from build123d import *

# Parameters (mm, degrees)
BOSS_EXTRUDE1_DEPTH = 2.2
SKETCH3_R           = 7.5
BOSS_EXTRUDE2_DEPTH = 2
BOSS_EXTRUDE3_DEPTH = 2.5
SKETCH5_W           = 12
SKETCH5_H           = 11
CUT_EXTRUDE1_DEPTH  = 7.7
SKETCH6_W           = 40
SKETCH6_H           = 20
SKETCH6_W_2         = 12
SKETCH6_H_2         = 11
BOSS_EXTRUDE4_DEPTH = 3
SKETCH7_R           = 1.75
CUT_EXTRUDE2_DEPTH  = 10.7
SKETCH8_R           = 3
CUT_EXTRUDE3_DEPTH  = 1.5
SKETCH9_W           = 40
SKETCH9_H           = 2.5
CUT_EXTRUDE4_DEPTH  = 10.7


with BuildPart() as part:
    # Sketch2 → Boss-Extrude1 (new body)
    with BuildSketch(Plane.XY):
        with BuildLine():
            Line((-5.830951895, -7.5), (5.830951895, -7.5))
            ThreePointArc((5.830951895, -7.5), (0, 9.5), (-5.830951895, -7.5))
        make_face()
    extrude(amount=-BOSS_EXTRUDE1_DEPTH)

    # Sketch3 → Boss-Extrude2 (add)
    with BuildSketch(Plane(origin=(0, 0, -2.2), x_dir=(-1, 0, 0), z_dir=(0, 0, -1))):
        Circle(SKETCH3_R)
    extrude(amount=BOSS_EXTRUDE2_DEPTH)

    # Sketch4 → Boss-Extrude3 (add)
    with BuildSketch(Plane(origin=(0, 0, -4.2), x_dir=(-1, 0, 0), z_dir=(0, 0, -1))):
        with BuildLine():
            Line((-5.830951895, -7.5), (5.830951895, -7.5))
            ThreePointArc((5.830951895, -7.5), (0, 9.5), (-5.830951895, -7.5))
        make_face()
    extrude(amount=BOSS_EXTRUDE3_DEPTH)

    # Sketch5 → Cut-Extrude1 (cut, through all)
    with BuildSketch(Plane(origin=(0, 0, -6.7), x_dir=(-1, 0, 0), z_dir=(0, 0, -1))):
        Rectangle(SKETCH5_W, SKETCH5_H)
    extrude(amount=-CUT_EXTRUDE1_DEPTH, mode=Mode.SUBTRACT)

    # Sketch6 → Boss-Extrude4 (add)
    with BuildSketch(Plane.XY):
        Rectangle(SKETCH6_W, SKETCH6_H)
        Rectangle(SKETCH6_W_2, SKETCH6_H_2, mode=Mode.SUBTRACT)
    extrude(amount=BOSS_EXTRUDE4_DEPTH)

    # Sketch7 → Cut-Extrude2 (cut, through all)
    with BuildSketch(Plane.XY.offset(3)):
        with Locations((-15, 0)):
            Circle(SKETCH7_R)
        with Locations((15, 0)):
            Circle(SKETCH7_R)
    extrude(amount=-CUT_EXTRUDE2_DEPTH, mode=Mode.SUBTRACT)

    # Sketch8 → Cut-Extrude3 (cut)
    with BuildSketch(Plane(origin=(0, 0, 0), x_dir=(-1, 0, 0), z_dir=(0, 0, -1))):
        with Locations((15, 0)):
            Circle(SKETCH8_R)
        with Locations((-15, 0)):
            Circle(SKETCH8_R)
    extrude(amount=-CUT_EXTRUDE3_DEPTH, mode=Mode.SUBTRACT)

    # Sketch9 → Cut-Extrude4 (cut, through all)
    with BuildSketch(Plane(origin=(0, 0, -6.7), x_dir=(-1, 0, 0), z_dir=(0, 0, -1))):
        with Locations((0, -8.75)):
            Rectangle(SKETCH9_W, SKETCH9_H)
    extrude(amount=-CUT_EXTRUDE4_DEPTH, mode=Mode.SUBTRACT)


solid = part.part
Verification items for the finished model (mm, model axes). A direction names the side the tool comes from. Give positions to 0.01 mm unless a question says otherwise; leave off trailing zeros. Loops run counter-clockwise (first coordinate to the right, second up) from the corner with the lowest first, then second, coordinate; pieces in that order, holes last.
1. Cross-section at D-D on y = 0. Count the separate pieces of the cut face and the enclosed holes in it, and give its area (3 significant figures).
Derived:
separate pieces: 4
enclosed holes: 0
area: 94.4 mm2
2. Release check for a two-part mould opening along Y. For faces 1 (the cylindrical face through (-0.1, 7.5, -3.2)), 2 (the cylindrical face through (0.33, 9.494, -1.085)), 3 (the flat face through (6, 0, -2)) record: +Y half, -Y half, draft (parallel to the pull), parting line (faces both ways), or undercut.
Derived:
face 1: +Y half
face 2: parting line
face 3: undercut
3. Tool access check on faces 4 (the cylindrical face through (0.1, -7.5, -3.2)), 5 (the flat face through (0, 5.5, -2)), 6 (the cylindrical face through (7.5, 0.1, -3.2)), 7 (the flat face through (13, 0, 1.5)). Record the directions out of +Z, -Z, +X, -X, +Y, -Y that give a thin tool (end or side, any length) a straight path to the whole face; none if there is none.
Derived:
face 4: -Y
face 5: +Z, -Z
face 6: +X
face 7: -Z
4. Go/stop test with flat-tipped pins: P1, Ø4.5, axis at x = -15, y = 0, coming from the -Z side; P2, Ø7, axis at x = -15, y = 0, coming from the +Z side; P3, Ø1.5, axis at y = -1.5, z = -3.5, coming from the -X side; P4, Ø6.5, axis at x = 15, y = -0.5, coming from the -Z side. Record where each tip stops, or that it passes through.
Derived:
P1: stops at z = 1.5
P2: stops at z = 3
P3: stops at x = -9.42
P4: stops at z = 0
5. Cross-section at C-C on z = 2.5. Record the cut outline in (x, y).
Derived:
outline: (-20, -7.5) - (20, -7.5) - (20, 10) - (-20, 10) - close; hole circle Ø3.5 at (-15, 0); hole (-6, -5.5) - (6, -5.5) - (6, 5.5) - (-6, 5.5) - close; hole circle Ø3.5 at (15, 0)
6. Cross-section at B-B on y = 8. Record the cut outline in (x, z), and give its area (3 significant figures).
Derived:
outline: (-20, 0) - (-5.12, 0) - (-5.12, -2.2) - (5.12, -2.2) - (5.12, 0) - (20, 0) - (20, 3) - (-20, 3) - close; (-5.12, -6.7) - (5.12, -6.7) - (5.12, -4.2) - (-5.12, -4.2) - close
area: 168 mm2
7. Cross-section at A-A on x = -15. Record the cut outline in (y, z).
Derived:
outline: (-7.5, 0) - (-3, 0) - (-3, 1.5) - (-1.75, 1.5) - (-1.75, 3) - (-7.5, 3) - close; (1.75, 1.5) - (3, 1.5) - (3, 0) - (10, 0) - (10, 3) - (1.75, 3) - close
8. Material ranges on probe 1 along X at (y, z) = (0, -3); probe 2 along Y at (x, z) = (-15, 2); probe 3 along X at (y, z) = (0, -1.5), recorded low to high.
Derived:
probe 1: x = -7.5 to -6, 6 to 7.5
probe 2: y = -7.5 to -1.75, 1.75 to 10
probe 3: x = -9.5 to -6, 6 to 9.5
